from build123d import *

# Parameters (mm, degrees)
F0_W          = 14.351
F0_H          = 34.925
F0_R          = 1.6256
F1_DEPTH      = 1.016
F1_DEPTH_BACK = 2.032
F2_R          = 1.9812
F3_DEPTH      = 6.35
F3_DEPTH_BACK = 12.7
F4_SIZE       = 1.524


with BuildPart() as f1:
    # F0 (on Top) → F1 (new body, two sides)
    with BuildSketch(Plane.XY) as f1_sk:
        Rectangle(F0_W, F0_H)
        with Locations((2.4257, -12.7127)):
            Circle(F0_R, mode=Mode.SUBTRACT)
        with Locations((2.4257, 12.7127)):
            Circle(F0_R, mode=Mode.SUBTRACT)
    extrude(amount=-F1_DEPTH)
    extrude(f1_sk.sketch, amount=F1_DEPTH_BACK)

    # F2 (on face) → F3 (join, two sides)
    with BuildSketch(Plane.XZ.offset(17.4625)) as f3_sk:
        with Locations((-5.5245, 1.9812)):
            Circle(F2_R)
    extrude(amount=F3_DEPTH)
    extrude(f3_sk.sketch, amount=-F3_DEPTH_BACK)

    # F4
    f4_edges = [f1.edges().sort_by_distance(p)[0] for p in [
        (-7.5057, -23.8125, 1.9812),
        (-6.120697, -4.7625, 3.870566),
    ]]
    chamfer(f4_edges, length=F4_SIZE)


solid = f1.part
Verification items for the finished model (mm, model axes). A direction names the side the tool comes from. Coordinates: 2 decimals unless noted, no trailing zeros. Order: outer loops, then holes, each group sorted by start corner. A loop starts at its lowest first (then second) coordinate and runs counter-clockwise, first axis right, second up. Notation, with made-up numbers: M -11,46 L 26,46 A25 cw 26,71 Z; hole C -30,53 d10. An arc over 180 degrees is marked long. Write each question's results on one line, items separated by ' | '.
1) Release check for a two-part mould opening along Y. For faces 1 (the face through (2.07, -14.3, 0.49)), 2 (the face through (-5.5, -23.812, 2)), 3 (the face through (7.176, 0, 0)) record: pulls with the +Y half, pulls with the -Y half, needs draft (parallel to the pull), parting line crosses it, or undercut.
Solved:
face 1: undercut | face 2: pulls with the -Y half | face 3: needs draft
2) Section check D-D on x = -1.5. Record the cut outline in (y, z).
Solved:
outline: M -17.46,-1.02 L 17.46,-1.02 L 17.46,2.03 L -17.46,2.03 Z
3) Section check B-B on z = -0.5. Record the cut outline in (x, y).
Solved:
outline: M -7.18,-17.46 L 7.18,-17.46 L 7.18,17.46 L -7.18,17.46 Z; hole C 2.43,-12.71 d3.25; hole C 2.43,12.71 d3.25
4) Access from +Z, -Z, +X, -X, +Y, -Y to the whole of each face (thin tool, end or side, straight path). Record for faces 4 (the face through (0, 0, -1.016)), 5 (the face through (-7.176, 0, 0)).
Solved:
face 4: -Z, +X, -X, +Y, -Y | face 5: -Z, -X, +Y
5) Section check C-C on y = -10. Record the cut outline in (x, z).
Solved:
outline: M -7.18,-1.02 L 7.18,-1.02 L 7.18,2.03 L -3.54,2.03 A1.98 ccw long -7.18,0.89 Z
6) Scan lines: line 1 along X through (y, z) = (-1, -0.2); line 2 along Y through (x, z) = (-1, 0.8); line 3 along Z through (x, y) = (-2, -10). Record each from-to range of solid material in increasing order. Write a range as [from, to].
Solved:
line 1: x = [-7.18, 7.18] | line 2: y = [-17.46, 17.46] | line 3: z = [-1.02, 2.03]
7) Gauge pin test, flat ends, axial feed: pin 1 Ø5 at (x, y) = (2.5, -10) entering from +Z; pin 2 Ø2 at (x, y) = (2.43, -12.71) entering from +Z; pin 3 Ø2.5 at (y, z) = (0.5, 1) entering from -X; pin 4 Ø1.5 at (x, z) = (-2.5, 1) entering from -Y. Record the tip position at first contact, or that the pin passes through.
Solved:
pin 1: stops at z = 2.03 | pin 2: passes through | pin 3: stops at x = -7.18 | pin 4: stops at y = -17.46
8) Section check A-A on x = 1.25. Record the cut outline in (y, z).
Solved:
outline: M -17.46,-1.02 L -13.84,-1.02 L -13.84,2.03 L -17.46,2.03 Z; M -11.59,-1.02 L 11.59,-1.02 L 11.59,2.03 L -11.59,2.03 Z; M 13.84,-1.02 L 17.46,-1.02 L 17.46,2.03 L 13.84,2.03 Z
